```python
from build123d import *

# Parameters (mm, degrees)
F0_W      = 12.7
F0_H      = 12.7
F1_DEPTH  = 12.7
F2_W      = 25.4
F2_H      = 25.4
F3_DEPTH  = 25.4
F5_DEPTH  = 25.4
F9_W      = 2.032
F9_H      = 12.7
F11_W     = 0.381
F11_H     = 0.5424337578
F11_H_2   = 0.2195662422
F13_DEPTH = 6.35


with BuildPart() as f1:
    # F0 (on Top) → F1 (new body)
    with BuildSketch(Plane.XY):
        with Locations((-6.35, 6.35)):
            Rectangle(F0_W, F0_H)
        with Locations((6.35, 6.35)):
            Rectangle(F0_W, F0_H)
        with Locations((-6.35, -6.35)):
            Rectangle(F0_W, F0_H)
        with Locations((6.35, -6.35)):
            Rectangle(F0_W, F0_H)
    extrude(amount=F1_DEPTH)

    # F2 (on face) → F3 (cut)
    with BuildSketch(Plane.XZ.offset(12.7)):
        with BuildLine():
            ThreePointArc((30.6605122425, 38.1), (-16.5933496542, 63.8823148345), (-12.7, 10.1934235175))
            Line((-12.7, 10.1934235175), (-12.7, 12.7))
            Line((-12.7, 12.7), (-12.7, 38.1))
            Line((-12.7, 38.1), (12.7, 38.1))
            Line((12.7, 38.1), (12.7, 12.7))
            Line((12.7, 12.7), (12.7, 10.1934235175))
            ThreePointArc((12.7, 10.1934235175), (25.7823148345, 21.5066503458), (30.6605122425, 38.1))
        make_face()
        with Locations((0, 25.4)):
            Rectangle(F2_W, F2_H)
        with BuildLine():
            Line((-12.7, 12.7), (-12.7, 10.1934235175))
            ThreePointArc((-12.7, 10.1934235175), (0, 7.4394877575), (12.7, 10.1934235175))
            Line((12.7, 10.1934235175), (12.7, 12.7))
            Line((12.7, 12.7), (-12.7, 12.7))
        make_face()
    extrude(amount=-F3_DEPTH, mode=Mode.SUBTRACT)

    # F4 (on face) → F5 (cut)
    with BuildSketch(Plane.YZ.offset(12.7)):
        Polygon((-12.7, 38.1), (-12.7, 10.1934235175), (0, 38.1), align=None)
        Polygon((12.7, 38.1), (0, 38.1), (12.7, 10.1934235175), align=None)
        with BuildLine():
            Line((12.7, 10.1934235175), (-12.7, 10.1934235175))
            ThreePointArc((-12.7, 10.1934235175), (-6.4975795911, 8.1358802828), (0, 7.4394877575))
            ThreePointArc((0, 7.4394877575), (6.4975795911, 8.1358802828), (12.7, 10.1934235175))
        make_face()
    extrude(amount=-F5_DEPTH, mode=Mode.SUBTRACT)

    # F9 (on offset) → F12 (revolve)
    with BuildSketch(Plane.XZ):
        Polygon((0, 17.9578), (2.032, 17.9578), (2.286, 17.9578), (0, 24.3078), align=None)
        with Locations((1.016, 11.6078)):
            Rectangle(F9_W, F9_H)
    revolve(axis=Axis((0, 0, 11.6078), (0, 0, 1)))

    # F11 (on offset) → F13 (cut)
    with BuildSketch(Plane(origin=(0, 0, 24.3078), x_dir=(1, 0, 0), z_dir=(0, 0, -1))):
        Polygon((0.381, 0.5424337578), (0.381, 2.286), (-0.381, 2.286), (-0.381, 0.5424337578), (0, 0.5424337578), align=None)
        Polygon((2.286, 0.5424337578), (0.381, 0.5424337578), (0.381, 0), (0.381, -0.2195662422), (2.286, -0.2195662422), align=None)
        with Locations((0.1905, 0.2712168789)):
            Rectangle(F11_W, F11_H)
        with Locations((-0.1905, 0.2712168789)):
            Rectangle(F11_W, F11_H)
        Polygon((-0.381, 0), (-0.381, 0.5424337578), (-2.286, 0.5424337578), (-2.286, -0.2195662422), (-0.381, -0.2195662422), align=None)
        with Locations((0.1905, -0.1097831211)):
            Rectangle(F11_W, F11_H_2)
        with Locations((-0.1905, -0.1097831211)):
            Rectangle(F11_W, F11_H_2)
        Polygon((0.381, -2.286), (0.381, -0.2195662422), (0, -0.2195662422), (-0.381, -0.2195662422), (-0.381, -2.286), align=None)
    extrude(amount=F13_DEPTH, mode=Mode.SUBTRACT)


solid = f1.part
```
Source: CAD feature listing. Evaluate the final solid. Frame: model axes, mm. A direction names the side the tool comes from. Coordinates: 2 decimals unless noted, no trailing zeros. Write each loop counter-clockwise with the first axis right and the second up, starting at its lowest first coordinate (ties: lowest second). Pieces come first, ordered by that corner, then holes. Notation, with made-up numbers: (-2, -16) -> (18, -16) arc R14 cw to (18, -7) -> close; hole circle Ø8 at (-9, 6.5). An arc over 180 degrees is marked (long way). Return JSON: item names as keys, results as strings. Group by question number.
1) Section query A-A, the plane x = 0. Return loops of the section in (y, z), plus the area to 3 significant figures.
2) Set-up query: faces 4 (the face through (-0.381, -1, 20)), 5 (the face through (-1, -0.542, 20)), 6 (the face through (0, 0, 17.958)), 7 (the face through (0, 12.7, 4)). Return all of +Z, -Z, +X, -X, +Y, -Y with unobstructed straight access to the full face (end or side cutting, diameter ignored); none if empty.
3) Ray query, line 1 along Y through (x, z) = (0, 16.25); line 2 along Z through (x, y) = (-10.75, 9). Return the intervals inside material, ascending.
4) Section query B-B, the plane y = -3.5. Return loops of the section in (x, z), plus the area to 3 significant figures.
5) Section query D-D, the plane x = 8.75. Return loops of the section in (y, z).
6) Section query C-C, the plane z = 13. Return loops of the section in (x, y).
7) Mould query, pull axis Z, two halves, no side actions, for faces 1 (the face through (-0.44, -1.984, 12.771)), 2 (the face through (-1.13, 1.07, 19.99)), 3 (the face through (0, 0, 0)). Classes: +Z half, -Z half, draft (parallel to the pull), parting line (faces both ways), or undercut.
8) Contact query for flat-ended pins moving along their axis: P1, Ø2, axis at y = 1.5, z = 20, coming from the +X side; P2, Ø0.5, axis at y = -1.5, z = 19.5, coming from the -X side; P3, Ø0.9, axis at x = 1, z = 20.5, coming from the +Y side. Output: stop coordinate, or through.
From the geometry:
{
 "1": {"outline": "(-12.7, 0) -> (12.7, 0) -> (12.7, 7.44) -> (2.03, 7.44) -> (2.03, 17.96) -> (-2.03, 17.96) -> (-2.03, 7.44) -> (-12.7, 7.44) -> close", "area": "232 mm²"},
 "2": {"face 4": "+Z, +Y, -Y", "face 5": "+Z, +X, -X", "face 6": "+Z", "face 7": "+Z, -Z, +X, -X, +Y"},
 "3": {"line 1": "-2.03 to 2.03", "line 2": "0 to 8.79"},
 "4": {"outline": "(-12.7, 0) -> (12.7, 0) -> (12.7, 7.64) -> (3.5, 7.64) arc R30.66 cw to (-3.5, 7.64) -> (-12.7, 7.64) -> close", "area": "193 mm²"},
 "5": {"outline": "(-12.7, 0) -> (12.7, 0) -> (12.7, 8.71) -> (8.75, 8.71) arc R30.66 cw to (-8.75, 8.71) -> (-12.7, 8.71) -> close"},
 "6": {"outline": "circle Ø4.06 at (0, 0)"},
 "7": {"face 1": "undercut", "face 2": "+Z half", "face 3": "-Z half"},
 "8": {"P1": "x = 1.62", "P2": "x = -1.23", "P3": "y = 1.32"}
}
